```python
from build123d import *

# Parameters (mm, degrees)
SKETCH1_W                 = 127
SKETCH1_H                 = 139.7
BOSS_EXTRUDE1_DEPTH       = 6.35
SKETCH5_W                 = 6.35
SKETCH5_H                 = 25.4
CUT_EXTRUDE4_DEPTH        = 6.35
SKETCH6_W                 = 25.4
SKETCH6_H                 = 6.35
CUT_EXTRUDE5_DEPTH        = 6.35
LPATTERN5_COUNT           = 3
LPATTERN5_PITCH           = 50.8
LPATTERN5_COUNT_DIR2      = 2
LPATTERN5_PITCH_DIR2      = 120.65
LPATTERN6_COUNT           = 3
LPATTERN6_PITCH           = 50.8
LPATTERN6_COUNT_DIR2      = 2
LPATTERN6_PITCH_DIR2      = 120.65
SKETCH7_W                 = 6.35
SKETCH7_H                 = 19.05
CUT_EXTRUDE6_DEPTH        = 6.35
SKETCH12_W                = 6.35
SKETCH12_H                = 12.7
CUT_EXTRUDE9_DEPTH        = 7.62
F_8_CLEARANCE_HOLE1_D     = 4.4958
F_8_CLEARANCE_HOLE1_DEPTH = 10.16
F_8_CLEARANCE_HOLE1_TIP   = 1.350674586
SKETCH11_R                = 1.143
SKETCH11_W                = 23.622
SKETCH11_H                = 23.622
CUT_EXTRUDE8_DEPTH        = 7.62


with BuildPart() as part:
    # Sketch1 → Boss-Extrude1 (new body)
    with BuildSketch(Plane.XY):
        with Locations((63.5, 69.85)):
            Rectangle(SKETCH1_W, SKETCH1_H)
    extrude(amount=BOSS_EXTRUDE1_DEPTH)

    # Sketch5 → Cut-Extrude4 (cut)
    with BuildSketch(Plane.XY.offset(6.35)):
        with Locations((3.175, 12.7)):
            Rectangle(SKETCH5_W, SKETCH5_H)
    cut_extrude4 = extrude(amount=-CUT_EXTRUDE4_DEPTH, mode=Mode.SUBTRACT)

    # Sketch6 → Cut-Extrude5 (cut)
    with BuildSketch(Plane.XY.offset(6.35)):
        with Locations((12.7, 3.175)):
            Rectangle(SKETCH6_W, SKETCH6_H)
    cut_extrude5 = extrude(amount=-CUT_EXTRUDE5_DEPTH, mode=Mode.SUBTRACT)

    # LPattern5: Cut-Extrude4 3 × 2
    with Locations(*[(j * LPATTERN5_PITCH_DIR2, i * LPATTERN5_PITCH, 0) for i in range(LPATTERN5_COUNT) for j in range(LPATTERN5_COUNT_DIR2) if (i, j) != (0, 0)]):
        add(cut_extrude4, mode=Mode.SUBTRACT)

    # LPattern6: Cut-Extrude5 3 × 2
    with Locations(*[(i * LPATTERN6_PITCH, j * LPATTERN6_PITCH_DIR2, 0) for i in range(LPATTERN6_COUNT) for j in range(LPATTERN6_COUNT_DIR2) if (i, j) != (0, 0)]):
        add(cut_extrude5, mode=Mode.SUBTRACT)

    # Sketch7 → Cut-Extrude6 (cut)
    with BuildSketch(Plane.XY.offset(6.35)):
        with Locations((3.175, 130.175)):
            Rectangle(SKETCH7_W, SKETCH7_H)
    extrude(amount=-CUT_EXTRUDE6_DEPTH, mode=Mode.SUBTRACT)

    # Sketch12 → Cut-Extrude9 (cut)
    with BuildSketch(Plane.XY.offset(6.35)):
        with Locations((123.825, 133.35)):
            Rectangle(SKETCH12_W, SKETCH12_H)
    extrude(amount=-CUT_EXTRUDE9_DEPTH, mode=Mode.SUBTRACT)

    # #8 Clearance Hole1
    with Locations(Plane.XY.offset(6.35)):
        with Locations((38.1, 123.825), (88.9, 123.825)):
            Hole(F_8_CLEARANCE_HOLE1_D / 2, depth=F_8_CLEARANCE_HOLE1_DEPTH)
            with Locations((0, 0, -(F_8_CLEARANCE_HOLE1_DEPTH + F_8_CLEARANCE_HOLE1_TIP / 2))):  # 118° drill point
                Cone(0, F_8_CLEARANCE_HOLE1_D / 2, F_8_CLEARANCE_HOLE1_TIP, mode=Mode.SUBTRACT)

    # Sketch11 → Cut-Extrude8 (cut)
    with BuildSketch(Plane.XY.offset(6.35)):
        with Locations((48.514, 70.739)):
            Circle(SKETCH11_R)
        with Locations((78.486, 70.739)):
            Circle(SKETCH11_R)
        with Locations((63.5, 70.739)):
            Rectangle(SKETCH11_W, SKETCH11_H)
    extrude(amount=-CUT_EXTRUDE8_DEPTH, mode=Mode.SUBTRACT)


solid = part.part
```
Geometry check sheet. Reference: the model listing, model coordinates, mm. A direction names the side the tool comes from. Give positions to 0.01 mm unless a question says otherwise; leave off trailing zeros. Write each loop counter-clockwise with the first axis right and the second up, starting at its lowest first coordinate (ties: lowest second). Pieces come first, ordered by that corner, then holes. Notation, with made-up numbers: (8.5, 2.25) - (12.5, 2.25) arc R33 ccw to (12.5, 41.25) - close; hole circle Ø10 at (35, 45.5). An arc over 180 degrees is marked (long way). Use a Markdown table: item, result.
Q1. Thickness scan on L1, parallel to Y at x = 65, z = 0.5; L2, parallel to Y at x = 38.1, z = 2.5; L3, parallel to Y at x = 117, z = 5.75. Record the ranges inside material, lowest first. Write a range as [from, to].
Computed:
| item | result |
|---|---|
| L1 | y = [6.35, 58.93], [82.55, 120.65], [127, 139.7] |
| L2 | y = [0, 121.58], [126.07, 139.7] |
| L3 | y = [6.35, 120.65], [127, 139.7] |
Q2. Section check C-C, the plane z = 4. Give the number of separate pieces and of enclosed holes in the cut face, then the cut area to 3 significant figures.
Computed:
| item | result |
|---|---|
| separate pieces | 1 |
| enclosed holes | 6 |
| area | 15,200 mm² |
Q3. Draft check along X on faces 1 (the face through (25.4, 124, 3)), 2 (the face through (89, 0, 3)), 3 (the face through (36.024, 122.964, 3.131)). Enter one of: pulls with the +X half, pulls with the -X half, needs draft (parallel to the pull), parting line crosses it, or undercut.
Computed:
| item | result |
|---|---|
| face 1 | pulls with the -X half |
| face 2 | needs draft |
| face 3 | undercut |
Q4. Go/stop test with flat-tipped pins: P1, Ø3, axis at y = 123, z = 2, coming from the +X side; P2, Ø3, axis at y = 125, z = 3, coming from the -X side; P3, Ø1.5, axis at y = 15.5, z = 0.5, coming from the +X side. Record where each tip stops, or that it passes through.
Computed:
| item | result |
|---|---|
| P1 | stops at x = 101.6 |
| P2 | stops at x = 25.4 |
| P3 | stops at x = 120.65 |
Q5. Section check B-B, the plane y = 10. Enter the section's corners in (x, z).
Computed:
| item | result |
|---|---|
| outline | (6.35, 0) - (120.65, 0) - (120.65, 6.35) - (6.35, 6.35) - close |
Q6. Section check A-A, the plane x = 38.1. Enter the section's corners in (y, z).
Computed:
| item | result |
|---|---|
| outline | (0, 0) - (121.58, 0) - (121.58, 6.35) - (0, 6.35) - close; (126.07, 0) - (139.7, 0) - (139.7, 6.35) - (126.07, 6.35) - close |
Q7. Set-up check for faces 4 (the face through (111, 6.35, 3)), 5 (the face through (3, 25.4, 3)), 6 (the face through (3, 76.2, 3)), 7 (the face through (50.8, 124, 3)): record each of +Z, -Z, +X, -X, +Y, -Y from which the full face is reachable in a straight line by a thin tool's end or side.
Computed:
| item | result |
|---|---|
| face 4 | +Z, -Z, +X, -Y |
| face 5 | +Z, -Z, -X, -Y |
| face 6 | +Z, -Z, -X |
| face 7 | +Z, -Z |
